Could you check a few things on this drawing? It's one solid part, dimensions in mm from its lowest x, y, z. Round coordinates to 2 decimals unless told otherwise and drop trailing zeros. Loops run counter-clockwise (first coordinate to the right, second up) from the corner with the lowest first, then second, coordinate; pieces in that order, holes last. Notation, with made-up numbers: (31, -21) -> (69, -21) arc R17 ccw to (69, -17) -> close; hole circle Ø1 at (-6, -26). An arc over 180 degrees is marked (long way). Write each question's results on one line, items separated by ' | '.
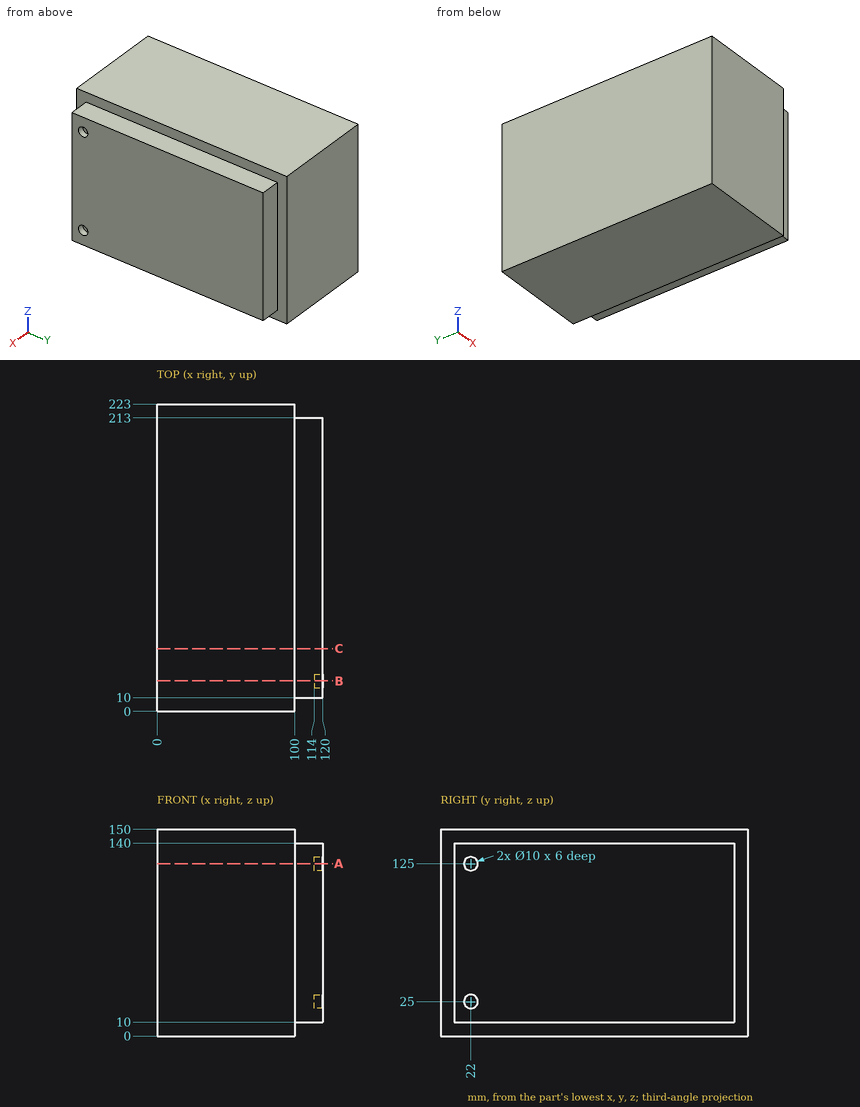
1) I want a section at A-A, the plane z = 125. Write out the boundary of the cut face in (x, y).
Model answer:
outline: (0, 0) -> (100, 0) -> (100, 10) -> (120, 10) -> (120, 17) -> (114, 17) -> (114, 27) -> (120, 27) -> (120, 213) -> (100, 213) -> (100, 223) -> (0, 223) -> close
2) I want a section at C-C, the plane y = 45.5. Write out the boundary of the cut face in (x, z).
Model answer:
outline: (0, 0) -> (100, 0) -> (100, 10) -> (120, 10) -> (120, 140) -> (100, 140) -> (100, 150) -> (0, 150) -> close
3) I'm going to push flat-ended pins straight in: pin 1 (22 mm diameter, centred on x = 114, z = 105, fed in from -Y); pin 2 (3 mm diameter, centred on y = 24, z = 124, fed in from +X); pin 3 (10 mm diameter, centred on y = 85, z = 109, fed in from -X); pin 4 (16 mm diameter, centred on x = 112.5, z = 75.5, fed in from +Y). Where does each tip first touch, or does it pass through?
Model answer:
pin 1: stops at y = 10 | pin 2: stops at x = 114 | pin 3: stops at x = 0 | pin 4: stops at y = 213
4) I want a section at B-B, the plane y = 22. Write out the boundary of the cut face in (x, z).
Model answer:
outline: (0, 0) -> (100, 0) -> (100, 10) -> (120, 10) -> (120, 20) -> (114, 20) -> (114, 30) -> (120, 30) -> (120, 120) -> (114, 120) -> (114, 130) -> (120, 130) -> (120, 140) -> (100, 140) -> (100, 150) -> (0, 150) -> close
5) I need wall thicknesses on line 1 (Y direction, x = 105.5, z = 44); line 2 (X direction, y = 133, z = 140.5); line 3 (Z direction, x = 101, y = 118.5). Which ranges of each line are inside material? Lowest first, please.
Model answer:
line 1: y = 10 to 213 | line 2: x = 0 to 100 | line 3: z = 10 to 140
